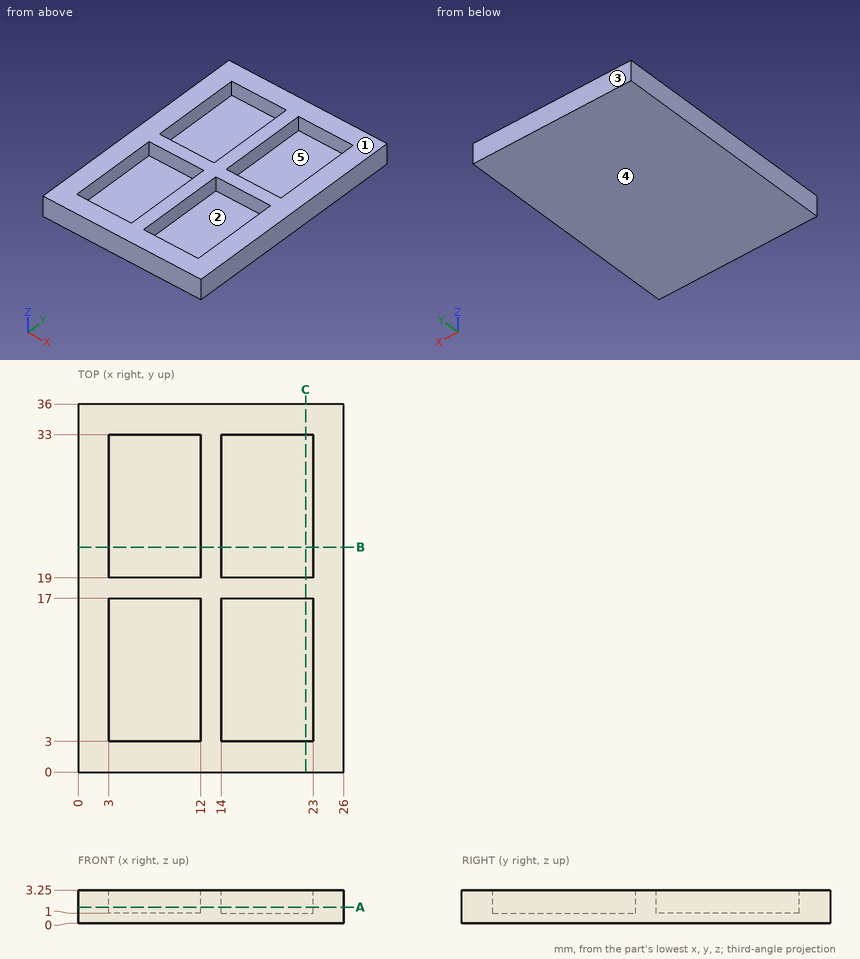
Geometry check sheet. Reference: drawing and pictorial views, mm from the part's lowest x, y, z. A direction names the side the tool comes from. Coordinates: 2 decimals unless noted, no trailing zeros. Loops run counter-clockwise (first coordinate to the right, second up) from the corner with the lowest first, then second, coordinate; pieces in that order, holes last.
1) Gauge pin test, flat end, axial feed: pin 1 (4.5 mm diameter, centred on x = 16.5, y = 13, fed in from +Z). Record the tip position at first contact, or that the pin passes through.
2) Release check for a two-part mould opening along Y. For the marked faces 1, 2 and 3 record: released by +Y, released by -Y, zero draft, split by the parting line, or undercut.
3) Material ranges on probe 1 along Y at (x, z) = (5, 1.1); probe 2 along X at (y, z) = (14.5, 1.35); probe 3 along Z at (x, y) = (20, 31), recorded low to high.
4) Sectioned sample at A-A (z = 1.6). Record the boundary of the cut face in (x, y).
5) Access from +Z, -Z, +X, -X, +Y, -Y to the whole of each face (thin tool, end or side, straight path). Record for the marked faces 4 and 5.
6) Sectioned sample at B-B (y = 22). Record the boundary of the cut face in (x, z), and give its area (3 significant figures).
7) Sectioned sample at C-C (x = 22.25). Record the boundary of the cut face in (y, z), and give its area (3 significant figures).
Check sheet entries:
1. pin 1: stops at z = 1
2. face 1: zero draft
2. face 2: undercut
2. face 3: released by +Y
3. probe 1: y = 0 to 3, 17 to 19, 33 to 36
3. probe 2: x = 0 to 3, 12 to 14, 23 to 26
3. probe 3: z = 0 to 1
4. outline: (0, 0) - (26, 0) - (26, 36) - (0, 36) - close; hole (3, 3) - (12, 3) - (12, 17) - (3, 17) - close; hole (3, 19) - (12, 19) - (12, 33) - (3, 33) - close; hole (14, 3) - (23, 3) - (23, 17) - (14, 17) - close; hole (14, 19) - (23, 19) - (23, 33) - (14, 33) - close
5. face 4: -Z, +X, -X, +Y, -Y
5. face 5: +Z
6. outline: (0, 0) - (26, 0) - (26, 3.25) - (23, 3.25) - (23, 1) - (14, 1) - (14, 3.25) - (12, 3.25) - (12, 1) - (3, 1) - (3, 3.25) - (0, 3.25) - close
6. area: 44.0 mm2
7. outline: (0, 0) - (36, 0) - (36, 3.25) - (33, 3.25) - (33, 1) - (19, 1) - (19, 3.25) - (17, 3.25) - (17, 1) - (3, 1) - (3, 3.25) - (0, 3.25) - close
7. area: 54.0 mm2
